Source: CAD feature listing. Evaluate the final solid. Frame: model axes, mm. Round coordinates to 2 decimals unless told otherwise and drop trailing zeros. Write item = value, one per line. Start each with the question number.
from build123d import *

# Parameters (mm, degrees)
EXTRUDE_1_DEPTH       = 330
EXTRUDE_3_DEPTH       = 330
PATTERN_CURVE_1_COUNT = 19
PATTERN_CURVE_1_PITCH = 10
SKETCH_3_R            = 2.1
SKETCH_3_R_2          = 2.6
SKETCH_3_R_3          = 1.6
SKETCH_3_R_4          = 1.3
CUT_EXTRUDE_1_DEPTH   = 8


with BuildPart() as part:
    # Эскиз1 → Вытянуть1 (new body)
    with BuildSketch(Plane.XY):
        with BuildLine():
            Line((0, 45), (3.52437539, 45))
            ThreePointArc((3.52437539, 45), (3.868987923, 44.862273656), (4.02375156, 44.524968808))
            Line((4.02375156, 44.524968808), (5.5, 15))
            Line((5.5, 15), (194.5, 15))
            Line((194.5, 15), (195.97624844, 44.524968808))
            ThreePointArc((195.97624844, 44.524968808), (196.131012077, 44.862273656), (196.47562461, 45))
            Line((196.47562461, 45), (200, 45))
            Line((200, 45), (200, 0))
            Line((200, 0), (0, 0))
            Line((0, 0), (0, 45))
        make_face()
    extrude(amount=EXTRUDE_1_DEPTH)

    # Эскиз2 → Вытянуть3 (add)
    with BuildSketch(Plane.XY.offset(330)):
        with BuildLine():
            Line((9.40067846, 44.428525275), (8, 15))
            Line((8, 15), (12, 15))
            Line((12, 15), (10.59932154, 44.428525275))
            ThreePointArc((10.59932154, 44.428525275), (10, 45), (9.40067846, 44.428525275))
        make_face()
    extrude_3 = extrude(amount=-EXTRUDE_3_DEPTH)

    # Кривая1: Вытянуть3 ×19
    with Locations(*[(i * PATTERN_CURVE_1_PITCH, 0, 0) for i in range(1, PATTERN_CURVE_1_COUNT)]):
        add(extrude_3)

    # Эскиз3 → Вырез-Вытянуть1 (cut)
    with BuildSketch(Plane.XZ):
        with Locations((9.5, 19.5)):
            Circle(SKETCH_3_R)
        with Locations((11.5, 151)):
            Circle(SKETCH_3_R)
        with Locations((16.5, 240)):
            Circle(SKETCH_3_R)
        with Locations((181.5, 210)):
            Circle(SKETCH_3_R)
        with Locations((188.5, 40)):
            Circle(SKETCH_3_R)
        with Locations((163.5, 130)):
            Circle(SKETCH_3_R)
        with Locations((63.5, 189)):
            Circle(SKETCH_3_R)
        with Locations((39.5, 79.5)):
            Circle(SKETCH_3_R_2)
        with Locations((114.5, 30)):
            Circle(SKETCH_3_R_3)
        with Locations((16.58, 183.75)):
            Circle(SKETCH_3_R_2)
        with Locations((84, 49)):
            Circle(SKETCH_3_R_4)
        with Locations((89, 89)):
            Circle(SKETCH_3_R_4)
        with Locations((61.5, 170)):
            Circle(SKETCH_3_R_4)
        with Locations((61.5, 210)):
            Circle(SKETCH_3_R_4)
        with Locations((108.5, 190)):
            Circle(SKETCH_3_R_4)
        with Locations((113.5, 220)):
            Circle(SKETCH_3_R)
    extrude(amount=-CUT_EXTRUDE_1_DEPTH, mode=Mode.SUBTRACT)


solid = part.part
(1) Cut plane A-A (y = 39). State how many separate pieces and enclosed holes the cut face has, and give its area (3 significant figures).
(2) Mould query, pull axis X, two halves, no side actions, for faces 1 (the face through (101, 13, 0)), 2 (the face through (161.31, 29.51, 167.31)). Classes: +X half, -X half, draft (parallel to the pull), parting line (faces both ways), or undercut.
(3) Pin query (flat end, axial travel): P1, Ø1.6, axis at x = 61.5, z = 210, coming from the -Y side; P2, Ø3, axis at x = 24.5, z = 167, coming from the +Y side. Return the tip coordinate at first contact, or that it passes through.
(4) Material intervals for line 1 along Z through (x, y) = (16, 5); line 2 along Z through (x, y) = (181.5, 6.25); line 3 along Z through (x, y) = (188.5, 6), sorted ascending. Write a range as from..to.
Solution:
q1.separate_pieces = 21
q1.enclosed_holes = 0
q1.area = 13,600 mm^2
q2.face_1 = draft
q2.face_2 = undercut
q3.P1 = 8
q3.P2 = 15
q4.line_1 = 0..181.22, 186.28..237.96, 242.04..330
q4.line_2 = 0..207.9, 212.1..330
q4.line_3 = 0..37.9, 42.1..330
